Answer from the drawing. Dimensions are ordinates in mm from the lowest x, y and z of the part. Coordinates: 2 decimals unless noted, no trailing zeros. Write each loop counter-clockwise with the first axis right and the second up, starting at its lowest first coordinate (ties: lowest second). Pieces come first, ordered by that corner, then holes.
(1) Find the intervals of material crossed by probe 1 along X at (y, z) = (0.8, 6.35) (3 decimals); probe 2 along Z at (x, y) = (5.08, 1.95); probe 3 along Z at (x, y) = (45, 0.2), in increasing order.
(2) Section B-B on z = 6.35 is taken. Write down the section's boundary in (x, y) (3 decimals), then the cut area to 3 significant figures.
(3) Given pin 1 (2.5 mm diameter, centred on x = 83.82, z = 6.35, fed in from +Y), flat-ended and moving along its own axis, determine where the tip first touches the part or whether it passes through.
(4) Section A-A on x = 44.45 is taken. Write down the section's boundary in (y, z) (3 decimals), then the cut area to 3 significant figures.
(5) Section C-C on y = 0.75 is taken. Write down the section's boundary in (x, z) (3 decimals).
(6) Section D-D on x = 5.08 is taken. Write down the section's boundary in (y, z), then the cut area to 3 significant figures.
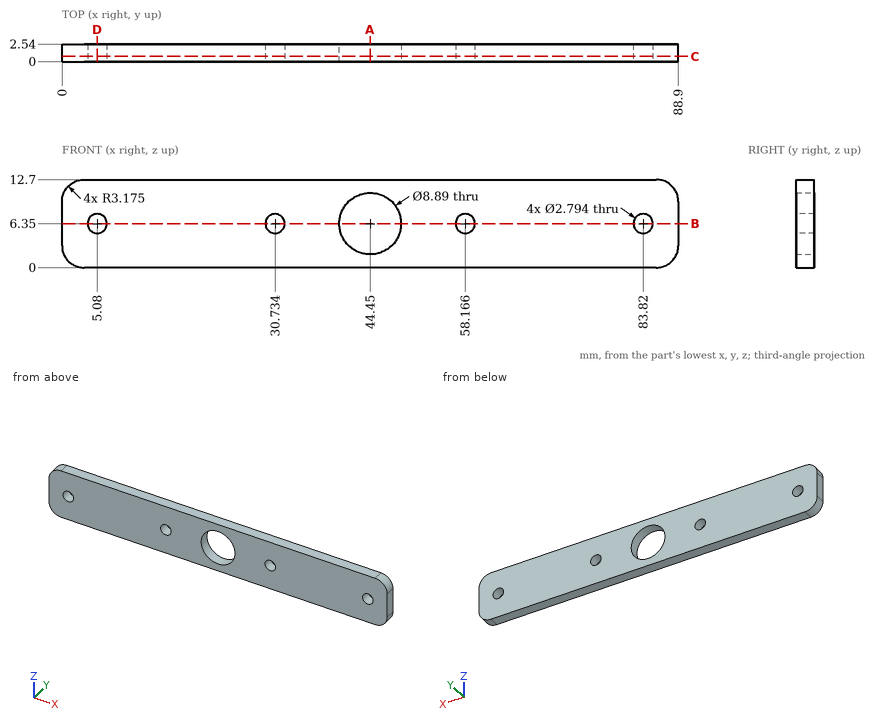
Response:
1. probe 1: x = 0 to 3.683, 6.477 to 29.337, 32.131 to 40.005, 48.895 to 56.769, 59.563 to 82.423, 85.217 to 88.9
1. probe 2: z = 0 to 4.95, 7.75 to 12.7
1. probe 3: z = 0 to 1.94, 10.76 to 12.7
2. outline: (0, 0) - (3.683, 0) - (3.683, 2.54) - (0, 2.54) - close; (6.477, 0) - (29.337, 0) - (29.337, 2.54) - (6.477, 2.54) - close; (32.131, 0) - (40.005, 0) - (40.005, 2.54) - (32.131, 2.54) - close; (48.895, 0) - (56.769, 0) - (56.769, 2.54) - (48.895, 2.54) - close; (59.563, 0) - (82.423, 0) - (82.423, 2.54) - (59.563, 2.54) - close; (85.217, 0) - (88.9, 0) - (88.9, 2.54) - (85.217, 2.54) - close
2. area: 175 mm2
3. pin 1: passes through
4. outline: (0, 0) - (2.54, 0) - (2.54, 1.905) - (0, 1.905) - close; (0, 10.795) - (2.54, 10.795) - (2.54, 12.7) - (0, 12.7) - close
4. area: 9.68 mm2
5. outline: (0, 3.175) arc R3.175 ccw to (3.175, 0) - (85.725, 0) arc R3.175 ccw to (88.9, 3.175) - (88.9, 9.525) arc R3.175 ccw to (85.725, 12.7) - (3.175, 12.7) arc R3.175 ccw to (0, 9.525) - close; hole circle Ø2.794 at (5.08, 6.35); hole circle Ø2.794 at (30.734, 6.35); hole circle Ø8.89 at (44.45, 6.35); hole circle Ø2.794 at (58.166, 6.35); hole circle Ø2.794 at (83.82, 6.35)
6. outline: (0, 0) - (2.54, 0) - (2.54, 4.95) - (0, 4.95) - close; (0, 7.75) - (2.54, 7.75) - (2.54, 12.7) - (0, 12.7) - close
6. area: 25.2 mm2
